Work out the finished part from the listing and answer in its coordinate system (mm). A direction names the side the tool comes from. Round coordinates to 2 decimals unless told otherwise and drop trailing zeros. Order: outer loops, then holes, each group sorted by start corner. A loop starts at its lowest first (then second) coordinate and runs counter-clockwise, first axis right, second up. Notation, with made-up numbers: M 10.5,-16.5 L 35.5,-16.5 A34 ccw 35.5,22.5 Z; hole C -37,-23.75 d7. An arc over 180 degrees is marked long. Return JSON: item names as keys, results as strings.
Autodesk Inventor part; units mm, degrees
ref_plane "YZ Plane" through (0, 0, 0) normal (1, 0, 0) x (0, 1, 0)
ref_plane "XZ Plane" through (0, 0, 0) normal (0, 1, 0) x (-1, 0, 0)
ref_plane "XY Plane" through (0, 0, 0) normal (0, 0, 1) x (1, 0, 0)
sketch "Sketch1" plane through (0, 0, 0) normal (1, 0, 0) x (0, 1, 0)
  line L0 (0, 17.9605) -> (17.9605, 0) construction
  line L1 (17.9605, 0) -> (0, -17.9605) construction
  line L2 (0, -17.9605) -> (-17.9605, 0) construction
  line L3 (-17.9605, 0) -> (0, 17.9605) construction
  line L4 (0, 17.9605) -> (0, -17.9605) construction
  line L5 (17.9605, 0) -> (-17.9605, 0) construction
  line L6 (0, 18.3816) -> (-18.3816, 0)
  line L7 (0, 18.3816) -> (18.3816, 0)
  line L8 (18.3816, 0) -> (0, -18.3816)
  line L9 (-18.3816, 0) -> (0, -18.3816)
  line L10 (0, 25.5658) -> (-25.5658, 0)
  line L11 (-25.5658, 0) -> (0, -25.5658)
  line L12 (0, -25.5658) -> (25.5658, 0)
  line L13 (25.5658, 0) -> (0, 25.5658)
  line L14 (-44.45, 0) -> (44.45, 0)
  line L15 (0, -44.45) -> (0, 44.45)
  line L16 (31.75, 31.75) -> (-31.75, 31.75)
  line L17 (-31.75, 31.75) -> (-31.75, -31.75)
  line L18 (-31.75, -31.75) -> (31.75, -31.75)
  line L19 (31.75, -31.75) -> (31.75, 31.75)
  line L20 (31.75, 31.75) -> (-31.75, -31.75) construction
  line L21 (-31.75, 31.75) -> (31.75, -31.75) construction
  point P0 (0, 0)
  point P1 (0, 0)
  point P2 (0, 0)
  point P3 (0, 0)
  point P4 (29.7157, 21.8287)
  point P5 (0, 0)
  dimension "d0" = 25.4
  dimension "d1" = 25.4
  dimension "d3" = 5.08
  dimension "d4" = 5.08
  dimension "d7" = 63.5
  dimension "d8" = 63.5
extrude "Extrusion1" add sketch "Sketch1" along normal mid plane 15.24 contours L15 L13 L14 L7 | L6 L14 L10 L15 | L9 L15 L11 L14 | L14 L12 L15 L8 | L15 L16 L19 L14 L13 | L10 L14 L17 L16 L15 | L11 L15 L18 L17 L14 | L14 L19 L18 L15 L12
equation "\"d4\" = d3"
equation "\"d8\" = d7"
properties part number "y_axis_mount" material "ABS Plastic"
Item 1: Find section C-C (z = -11). Determine the outline of the cut face in (x, y).
Output:
{"outline": "M -7.62,-31.75 L 7.62,-31.75 L 7.62,-7.38 L -7.62,-7.38 Z; M -7.62,7.38 L 7.62,7.38 L 7.62,31.75 L -7.62,31.75 Z"}
Item 2: This flat-tipped pin is pushed along its axis until it touches: pin 1 (10 mm diameter, centred on y = 8.5, z = -1, fed in from +X). Where does it stop, or does it pass through?
Output:
{"pin 1": "passes through"}
Item 3: Find section A-A (y = 7). Determine the outline of the cut face in (x, z).
Output:
{"outline": "M -7.62,-31.75 L 7.62,-31.75 L 7.62,-11.38 L -7.62,-11.38 Z; M -7.62,11.38 L 7.62,11.38 L 7.62,31.75 L -7.62,31.75 Z"}
Item 4: The mould has two halves that part along Y. Classify faces 3 (the flat face through (0, 0, 31.75)), 4 (the flat face through (-0.11, 9.32, -9.06)), 5 (the flat face through (0, 31.75, 0)): pulls with the +Y half, pulls with the -Y half, needs draft (parallel to the pull), parting line crosses it, or undercut.
Output:
{"face 3": "needs draft", "face 4": "undercut", "face 5": "pulls with the +Y half"}
Item 5: Which of the six approach directions +Z, -Z, +X, -X, +Y, -Y give full straight-line access (tool end or side, diameter ignored) to faces 1 (the flat face through (-0.11, -9.06, 9.32)), 2 (the flat face through (7.62, 14, 8))?
Output:
{"face 1": "+X, -X", "face 2": "+Z, -Z, +X, +Y, -Y"}
Item 6: Consider line 1 along Y through (x, z) = (3.25, -13.5); line 2 along Y through (x, z) = (3.25, -15.5); line 3 along Z through (x, y) = (5.25, 10.5). Determine where each line is inside the solid, lowest interval first. Write a range as [from, to].
Output:
{"line 1": "y = [-31.75, -4.88], [4.88, 31.75]", "line 2": "y = [-31.75, -2.88], [2.88, 31.75]", "line 3": "z = [-31.75, -7.88], [7.88, 31.75]"}
Item 7: Find section B-B (x = -0.75). Determine the outline of the cut face in (y, z), plus the area to 3 significant figures.
Output:
{"outline": "M -31.75,-31.75 L 31.75,-31.75 L 31.75,31.75 L -31.75,31.75 Z; hole M -18.38,0 L 0,-18.38 L 18.38,0 L 0,18.38 Z", "area": "3,360 mm^2"}
